Can you work these out from the drawing? Everything is in mm from the part's minimum corner. Coordinates: 2 decimals unless noted, no trailing zeros. Loops run counter-clockwise (first coordinate to the right, second up) from the corner with the lowest first, then second, coordinate; pieces in that order, holes last. Notation, with made-up numbers: M 53.25,-19.5 L 65.25,-19.5 A16 ccw 65.25,3.5 Z; hole C -20.5,-18.75 d7. An arc over 180 degrees is marked long. Write each question's results on one line, items separated by ' | '.
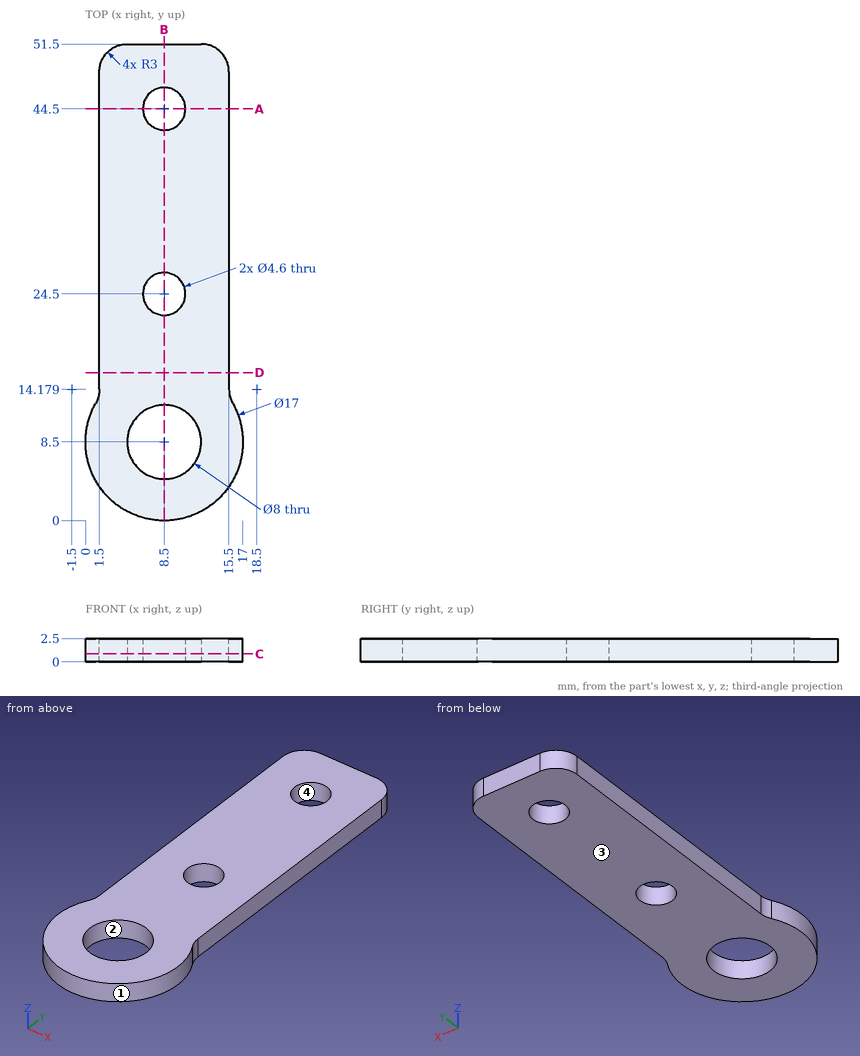
(1) Imagine slicing it at B-B, the plane x = 8.5. List the corners of the cut face in (y, z) for me.
Reported:
outline: M 0,0 L 4.5,0 L 4.5,2.5 L 0,2.5 Z; M 12.5,0 L 22.2,0 L 22.2,2.5 L 12.5,2.5 Z; M 26.8,0 L 42.2,0 L 42.2,2.5 L 26.8,2.5 Z; M 46.8,0 L 51.5,0 L 51.5,2.5 L 46.8,2.5 Z
(2) Will these pins go through, and if not, where does the flat tip stop? P1, Ø1.2, axis at y = 36.5, z = 1.5, coming from the +X side; P2, Ø3.5, axis at x = 8.5, y = 44.5, coming from the -Z side.
Reported:
P1: stops at x = 15.5 | P2: passes through
(3) Please list where these lines run through material, in increasing order: probe 1 along Y at (x, z) = (8.5, 0.6); probe 2 along Y at (x, z) = (8, 2.45) (1 decimal); probe 3 along X at (y, z) = (20.5, 2.35). Write a range as from..to.
Reported:
probe 1: y = 0..4.5, 12.5..22.2, 26.8..42.2, 46.8..51.5 | probe 2: y = 0..4.5, 12.5..22.3, 26.7..42.3, 46.7..51.5 | probe 3: x = 1.5..15.5
(4) Imagine slicing it at D-D, the plane y = 16. List the corners of the cut face in (x, z) for me.
Reported:
outline: M 1.5,0 L 15.5,0 L 15.5,2.5 L 1.5,2.5 Z
(5) Imagine slicing it at C-C, the plane z = 0.85. List the corners of the cut face in (x, y) for me.
Reported:
outline: M 1.11,12.7 A8.5 ccw long 15.89,12.7 A3 cw 15.5,14.18 L 15.5,48.5 A3 ccw 12.5,51.5 L 4.5,51.5 A3 ccw 1.5,48.5 L 1.5,14.18 A3 cw Z; hole C 8.5,8.5 d8; hole C 8.5,24.5 d4.6; hole C 8.5,44.5 d4.6
(6) If we mould it in two halves opening along X, with no side actions, what happens to the marked faces 1, 2, 3 and 4? For each: released by +X, released by -X, zero draft, split by the parting line, or undercut.
Reported:
face 1: split by the parting line | face 2: undercut | face 3: zero draft | face 4: undercut
(7) Imagine slicing it at A-A, the plane y = 44.5. List the corners of the cut face in (x, z) for me, and give its area (3 significant figures).
Reported:
outline: M 1.5,0 L 6.2,0 L 6.2,2.5 L 1.5,2.5 Z; M 10.8,0 L 15.5,0 L 15.5,2.5 L 10.8,2.5 Z | area: 23.5 mm2
